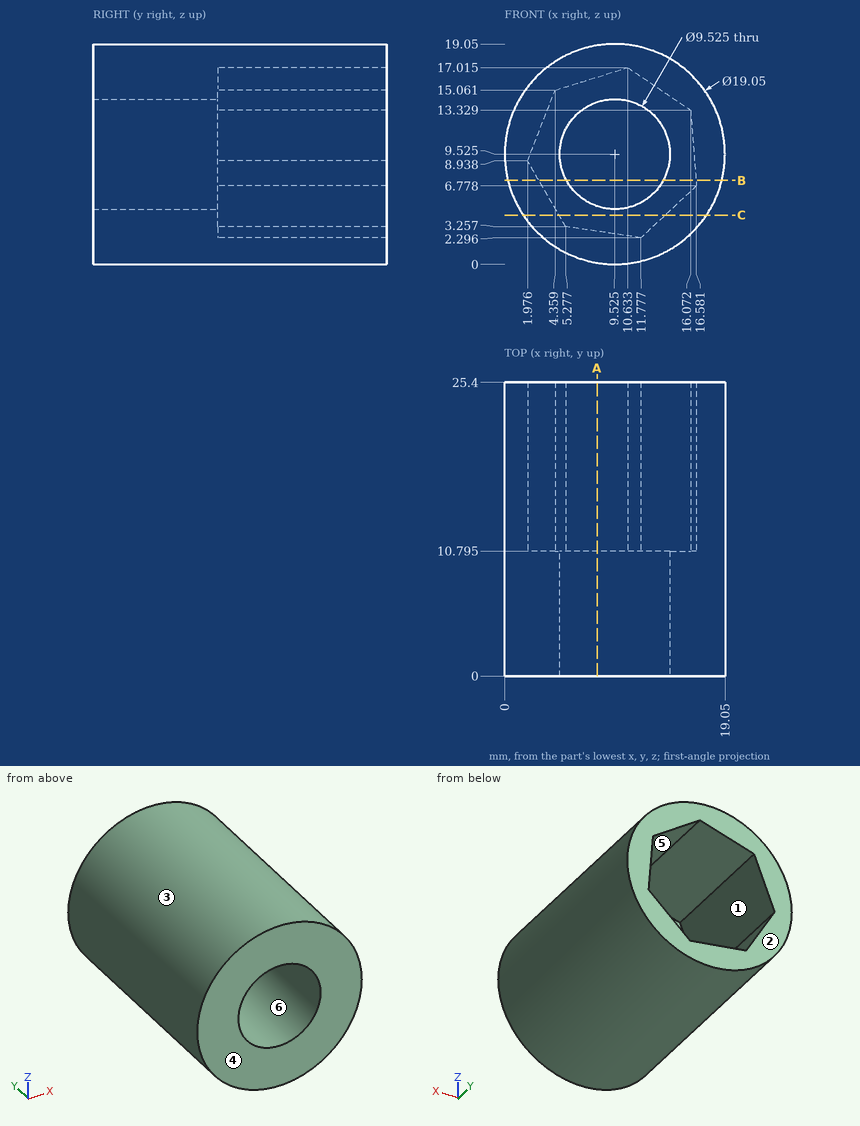
For this review, use the dimensioned drawing (mm, ordinates from the lowest corner) and the shaded views. A direction names the side the tool comes from. Coordinates: 2 decimals unless noted, no trailing zeros. Loops run counter-clockwise (first coordinate to the right, second up) from the corner with the lowest first, then second, coordinate; pieces in that order, holes last. Notation, with made-up numbers: (-37.5, 45) -> (-32.5, 45) arc R22 ccw to (-32.5, 60) -> close; hole circle Ø6 at (-22.5, 52). An arc over 180 degrees is marked (long way). Return JSON: item names as keys, results as strings. Group by question number.
(1) Consider section C-C, the plane z = 4.25. Give the boundary of the cut face in (x, y) (1 decimal).
(2) Mouldability with a two-part tool opening along Z and no side actions: class the marked faces 3, 4, 5 and 6 as pulls with the +Z half, pulls with the -Z half, needs draft (parallel to the pull), parting line crosses it, or undercut.
(3) To check wall thickness, follow L1, parallel to X at y = 1.5, z = 9.5; L2, parallel to Z at x = 10.75, y = 21 (1 decimal); L3, parallel to Y at x = 14.5, z = 9 (1 decimal). State the ranges of each line that lie inside material, in increasing order.
(4) Consider section B-B, the plane z = 7.25. Give the boundary of the cut face in (x, y) (1 decimal).
(5) For pin 1 Ø1 at (x, y) = (12.5, 14) entering from -Z; pin 2 Ø2 at (y, z) = (5.5, 13) entering from +X; pin 3 Ø4 at (y, z) = (20, 4) entering from +X, all flat-tipped, find the tip position at first contact; note any pin that passes through.
(6) Consider section A-A, the plane x = 8. Give the boundary of the cut face in (y, z) (1 decimal), plus the area to 3 significant figures.
(7) Tool access review of the marked faces 1 and 2: name each direction out of +Z, -Z, +X, -X, +Y, -Y from which nothing blocks a thin tool from reaching the whole face with its end or side.
Results below:
{
 "1": {"outline": "(1.6, 0) -> (17.5, 0) -> (17.5, 25.4) -> (13.9, 25.4) -> (13.9, 10.8) -> (4.7, 10.8) -> (4.7, 25.4) -> (1.6, 25.4) -> close"},
 "2": {"face 3": "parting line crosses it", "face 4": "needs draft", "face 5": "undercut", "face 6": "undercut"},
 "3": {"L1": "x = 0 to 4.76, 14.29 to 19.05", "L2": "z = 0.1 to 2.4, 16.9 to 19", "L3": "y = 0 to 10.8"},
 "4": {"outline": "(0.3, 0) -> (5.3, 0) -> (5.3, 10.8) -> (3, 10.8) -> (3, 25.4) -> (0.3, 25.4) -> close; (13.7, 0) -> (18.8, 0) -> (18.8, 25.4) -> (16.5, 25.4) -> (16.5, 10.8) -> (13.7, 10.8) -> close"},
 "5": {"pin 1": "stops at z = 0.33", "pin 2": "stops at x = 18.72", "pin 3": "stops at x = 18.37"},
 "6": {"outline": "(0, 0.1) -> (25.4, 0.1) -> (25.4, 2.9) -> (10.8, 2.9) -> (10.8, 5) -> (0, 5) -> close; (0, 14) -> (10.8, 14) -> (10.8, 16.2) -> (25.4, 16.2) -> (25.4, 18.9) -> (0, 18.9) -> close", "area": "185 mm2"},
 "7": {"face 1": "+Y", "face 2": "+Z, -Z, +X, -X, +Y"}
}
